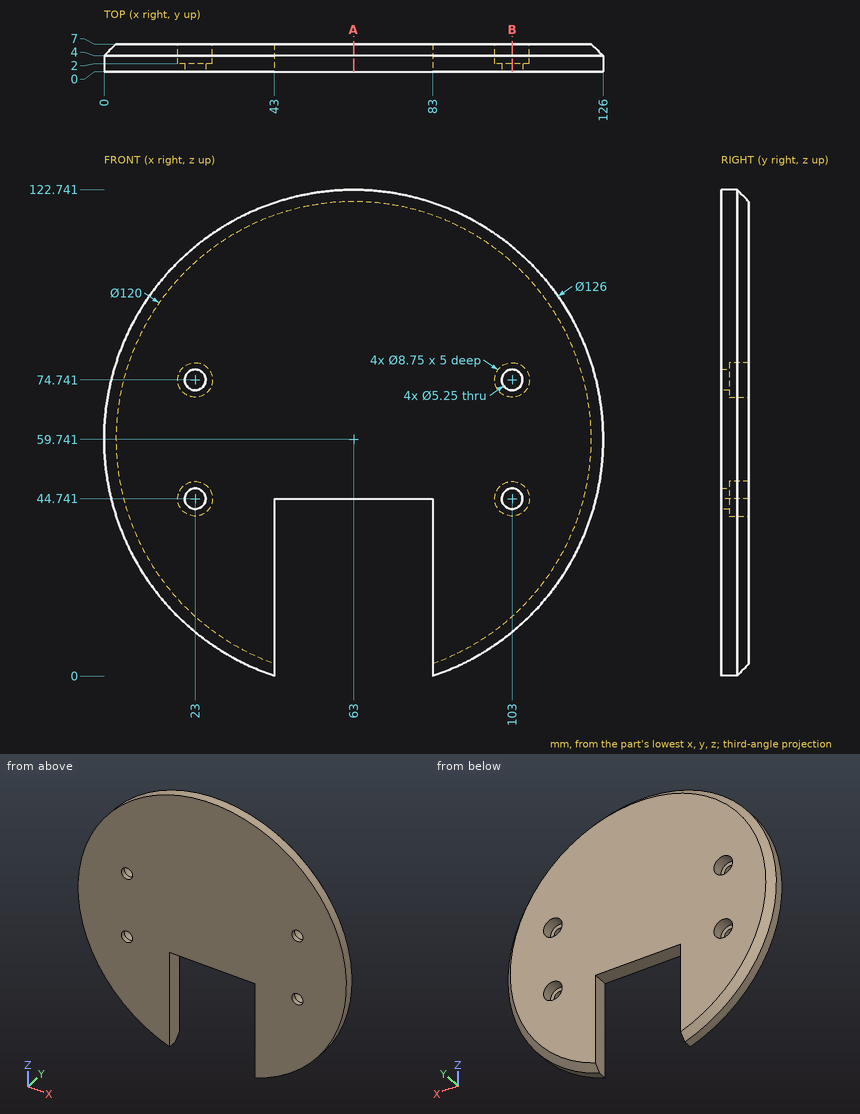
For this review, use the dimensioned drawing (mm, ordinates from the lowest corner) and the shaded views. Round coordinates to 2 decimals unless told otherwise and drop trailing zeros. Order: outer loops, then holes, each group sorted by start corner. A loop starts at its lowest first (then second) coordinate and runs counter-clockwise, first axis right, second up. Notation, with made-up numbers: M -9,-20 L 14,-20 A10 ccw 14,-5 Z; hole C 55.25,5 d2. An arc over 180 degrees is marked long. Use a Markdown table: item, result. Add a question column.
Item 1: Add section A-A, the plane x = 63. Give the boundary of the cut face in (y, z), then the cut area to 4 significant figures.
Item 2: Add section B-B, the plane x = 103. State how many separate pieces and enclosed holes the cut face has, then the cut area to 3 significant figures.
Item 3: To check wall thickness, follow line 1 along X through (y, z) = (2.5, 71) (1 decimal); line 2 along Z through (x, y) = (103, 1.1); line 3 along X through (y, z) = (5.5, 41) (1 decimal). State the ranges of each line that lie inside material, in increasing order.
Item 4: Insertion check: pin 1 (2 mm diameter, centred on x = 27.5, z = 13, fed in from -Y); pin 2 (3 mm diameter, centred on y = 6, z = 56.5, fed in from +X); pin 3 (4.5 mm diameter, centred on x = 23, z = 74.74, fed in from -Y); pin 4 (7 mm diameter, centred on x = 103, z = 44.74, fed in from +Y). Each pin has a flat end and moves straight along its axis. Give the tip position at first contact, or say it passes through.
Geometry results:
| question | item | result |
|---|---|---|
| 1 | outline | M 0,44.74 L 7,44.74 L 7,119.74 L 4,122.74 L 0,122.74 Z |
| 1 | area | 541.5 mm² |
| 2 | separate pieces | 3 |
| 2 | enclosed holes | 0 |
| 2 | area | 561 mm² |
| 3 | line 1 | x = 1 to 20.7, 25.3 to 100.7, 105.3 to 125 |
| 3 | line 2 | z = 11.07 to 42.12, 47.37 to 72.12, 77.37 to 108.41 |
| 3 | line 3 | x = 4.4 to 20.7, 25.3 to 43, 83 to 100.7, 105.3 to 121.6 |
| 4 | pin 1 | stops at y = 0 |
| 4 | pin 2 | stops at x = 125.42 |
| 4 | pin 3 | passes through |
| 4 | pin 4 | stops at y = 2 |
